Here's how the part is built. I have some questions about the finished solid (model axes, mm). Face numbers are marked on the shaded views. Give positions to 0.01 mm unless a question says otherwise; leave off trailing zeros. Write each loop counter-clockwise with the first axis right and the second up, starting at its lowest first coordinate (ties: lowest second). Pieces come first, ordered by that corner, then holes. Notation, with made-up numbers: (48, 68.5) - (104, 68.5) arc R32 cw to (104, 101.5) - close; hole circle Ø6 at (85, 81.5). An arc over 180 degrees is marked (long way). Write each question's results on one line, items separated by ' | '. Start each with the question number.
Item 1: Please list where these lines run through material, in increasing order: line 1 along X through (y, z) = (-142, 21.5) (3 decimals); line 2 along Y through (x, z) = (14.5, 25) (3 decimals); line 3 along Y through (x, z) = (16.25, 214.5) (1 decimal).
Item 2: Suppose I cut it at B-B on y = 9. List the corners of the cut face in (x, z) for me (3 decimals), then the cut area to 3 significant figures.
Item 3: Suppose I cut it at A-A on x = 14.75. List the corners of the cut face in (y, z) for me (3 decimals).
Item 4: We'd pull the mould along Y, two halves only. Please class the marked faces 1, 2, 3 and 4: +Y half, -Y half, draft (parallel to the pull), parting line (faces both ways), or undercut.
Item 5: Suppose I cut it at D-D on z = 173. List the corners of the cut face in (x, y) for me (3 decimals).
Item 6: Suppose I cut it at C-C on z = 279. List the corners of the cut face in (x, y) for me (3 decimals).
Item 7: Will these pins go through, and if not, where does the flat tip stop? P1, Ø1, axis at x = 21, y = -94.5, coming from the +Z side; P2, Ø1.5, axis at x = 9, z = 119.5, coming from the -Y side; P3, Ø1.5, axis at x = 6.5, z = 250, coming from the -Y side.
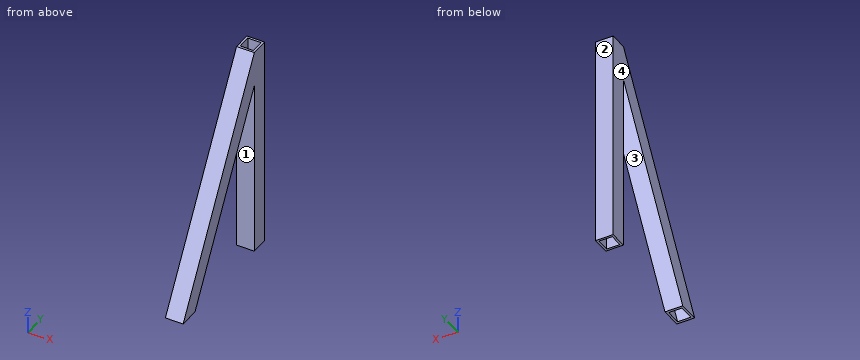
```python
from build123d import *

# Parameters (mm, degrees)
SKETCH1_W           = 25.4
SKETCH1_H           = 25.4
SKETCH1_W_2         = 19.05
SKETCH1_H_2         = 19.05
BOSS_EXTRUDE1_DEPTH = 304.8
SKETCH2_W           = 25.4
SKETCH2_H           = 50.8
SKETCH2_W_2         = 19.05
SKETCH2_H_2         = 38.1
SKETCH4_W           = 26.690109794
SKETCH4_H           = 109.792846898
CUT_EXTRUDE1_DEPTH  = 375.380835514


with BuildPart() as part:
    # Sketch1 → Boss-Extrude1 (new body)
    with BuildSketch(Plane.XY):
        with Locations((12.7, 12.7)):
            Rectangle(SKETCH1_W, SKETCH1_H)
        with Locations((12.7, 12.7)):
            Rectangle(SKETCH1_W_2, SKETCH1_H_2, mode=Mode.SUBTRACT)
    extrude(amount=BOSS_EXTRUDE1_DEPTH)

    # Sweep1: sweep along a path in Sketch3
    with BuildLine(Plane(origin=(25.4, 0, 0), x_dir=(0, 0, -1), z_dir=(1, 0, 0))) as sweep1_path:
        Line((-279.4, 0), (50.555678842, -190.5))
    # Sketch2 → Sweep1 (sweep)
    with BuildSketch(Plane.XZ):
        with Locations((12.7, 279.4)):
            Rectangle(SKETCH2_W, SKETCH2_H)
        with Locations((12.7, 279.4)):
            Rectangle(SKETCH2_W_2, SKETCH2_H_2, mode=Mode.SUBTRACT)
    sweep(path=sweep1_path.line)

    # Sketch4 → Cut-Extrude1 (cut, through all)
    with BuildSketch(Plane(origin=(0, 25.4, 0), x_dir=(1, 0, 0), z_dir=(0, 1, 0))):
        with Locations((13.345054897, 54.896423449)):
            Rectangle(SKETCH4_W, SKETCH4_H)
    extrude(amount=-CUT_EXTRUDE1_DEPTH, mode=Mode.SUBTRACT)


solid = part.part
```
Checked values:
1) line 1: x = 0 to 3.175, 22.225 to 25.4 | line 2: y = -161.543 to -157.876, -135.879 to -132.213, 0 to 3.175, 22.225 to 25.4 | line 3: y = -52.1 to -48.5, -26.5 to -22.8, 0 to 3.2, 22.2 to 25.4
2) outline: (0, 0) - (3.175, 0) - (3.175, 304.8) - (0, 304.8) - close; (22.225, 0) - (25.4, 0) - (25.4, 304.8) - (22.225, 304.8) - close | area: 1,940 mm^2
3) outline: (-175.976, 0) - (-172.31, 0) - (0, 298.45) - (0, 260.35) - (-150.313, 0) - (-146.647, 0) - (0, 254) - (0, 0) - (3.175, 0) - (3.175, 304.8) - (0, 304.8) - close; (22.225, 0) - (25.4, 0) - (25.4, 304.8) - (22.225, 304.8) - close
4) face 1: undercut | face 2: +Y half | face 3: undercut | face 4: draft
5) outline: (0, -76.095) - (25.4, -76.095) - (25.4, -46.765) - (0, -46.765) - close; (0, 0) - (25.4, 0) - (25.4, 25.4) - (0, 25.4) - close; hole (3.175, -72.429) - (22.225, -72.429) - (22.225, -50.432) - (3.175, -50.432) - close; hole (3.175, 3.175) - (22.225, 3.175) - (22.225, 22.225) - (3.175, 22.225) - close
6) outline: (0, -14.896) - (25.4, -14.896) - (25.4, 25.4) - (0, 25.4) - close; hole (3.175, -11.229) - (22.225, -11.229) - (22.225, 0) - (3.175, 0) - close; hole (3.175, 3.175) - (22.225, 3.175) - (22.225, 22.225) - (3.175, 22.225) - close
7) P1: stops at z = 141.99 | P2: stops at y = -107.42 | P3: stops at y = -32.07
